Print and shaded views of the part. All mm, measured from the part's lowest x, y and z. Coordinates: 2 decimals unless noted, no trailing zeros. Loops run counter-clockwise (first coordinate to the right, second up) from the corner with the lowest first, then second, coordinate; pieces in that order, holes last. Notation, with made-up numbers: M 42,7 L 72,7 A18 cw 72,17 Z; hole C 16,56.5 d9. An arc over 180 degrees is marked long. Answer as CSV lines item,"result". Start each with the question number.
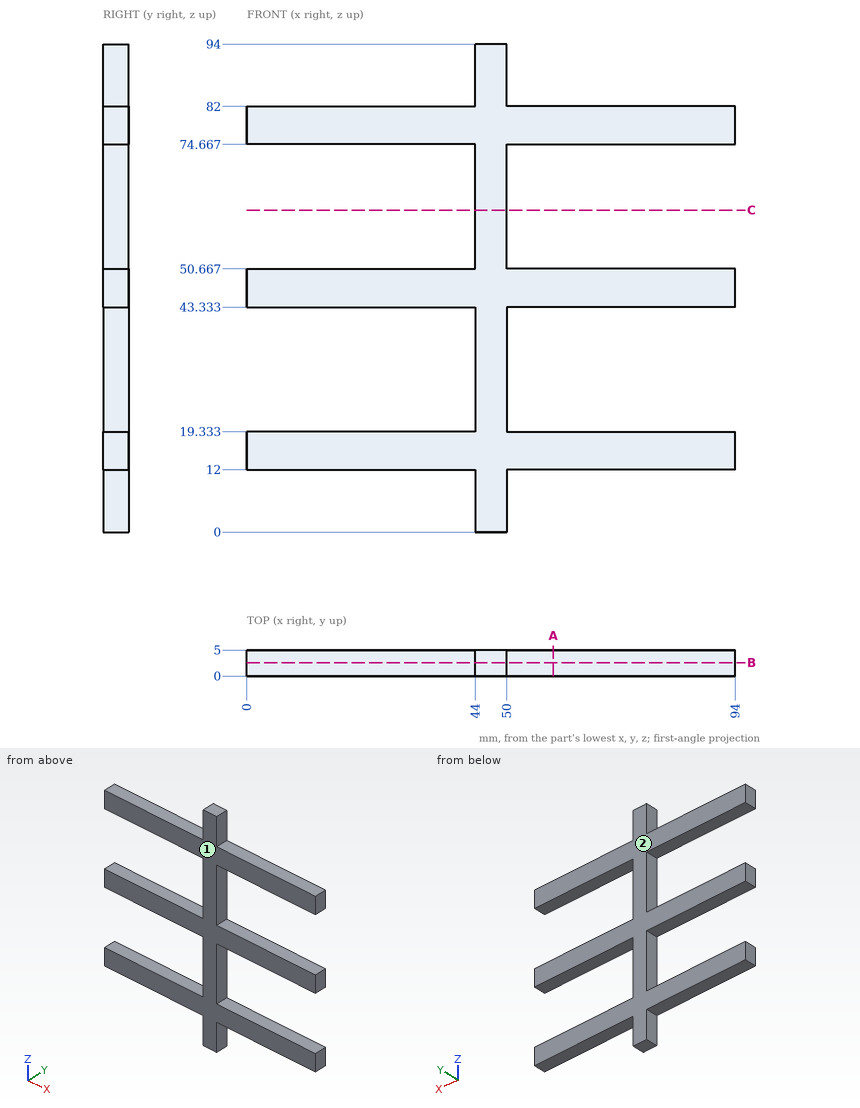
Q1. Slice it at C-C, the plane z = 62. Write the cut outline in (x, y).
Q2. Two-plate mould, pull along Y, no slides. Class the marked faces 1 and 2: +Y half, -Y half, draft (parallel to the pull), parting line (faces both ways), or undercut.
Q3. Wall check: L1, parallel to Z at x = 33.5, y = 1.15; L2, parallel to X at y = 4.45, z = 88.5. Give the ranges that are in metal, low to high.
Q4. Slice it at A-A, the plane x = 59. Write the cut outline in (y, z), and give its area (3 significant figures).
Q5. Flat gauge pins, fed straight in: P1, Ø1.5, axis at x = 42, y = 2.5, coming from the -Z side; P2, Ø2.5, axis at x = 74.5, y = 1.5, coming from the +Z side; P3, Ø2.5, axis at y = 3.5, z = 66.5, coming from the -X side. Where does each tip first touch, or does it go through?
Q6. Slice it at B-B, the plane y = 2.6. Write the cut outline in (x, z).
Solved:
1,outline,"M 44,0 L 50,0 L 50,5 L 44,5 Z"
2,face 1,"-Y half"
2,face 2,"+Y half"
3,L1,"z = 12 to 19.33, 43.33 to 50.67, 74.67 to 82"
3,L2,"x = 44 to 50"
4,outline,"M 0,12 L 5,12 L 5,19.33 L 0,19.33 Z; M 0,43.33 L 5,43.33 L 5,50.67 L 0,50.67 Z; M 0,74.67 L 5,74.67 L 5,82 L 0,82 Z"
4,area,"110 mm2"
5,P1,"stops at z = 12"
5,P2,"stops at z = 82"
5,P3,"stops at x = 44"
6,outline,"M 0,12 L 44,12 L 44,0 L 50,0 L 50,12 L 94,12 L 94,19.33 L 50,19.33 L 50,43.33 L 94,43.33 L 94,50.67 L 50,50.67 L 50,74.67 L 94,74.67 L 94,82 L 50,82 L 50,94 L 44,94 L 44,82 L 0,82 L 0,74.67 L 44,74.67 L 44,50.67 L 0,50.67 L 0,43.33 L 44,43.33 L 44,19.33 L 0,19.33 Z"
